Geometry check sheet. Reference: the model listing, model coordinates, mm. A direction names the side the tool comes from. Give positions to 0.01 mm unless a question says otherwise; leave off trailing zeros. Write each loop counter-clockwise with the first axis right and the second up, starting at its lowest first coordinate (ties: lowest second). Pieces come first, ordered by that corner, then holes. Notation, with made-up numbers: (27, 44) - (82, 44) arc R15 ccw to (82, 64) - close; hole circle Ø1 at (2, 4.5). An arc over 180 degrees is marked (long way). Write item = value, one per line. Start each with the question number.
(1) Section check D-D, the plane x = 12.5. Enter the section's corners in (y, z), plus the area to 3 significant figures.
(2) Depth check by flat-ended pin: pin 1 Ø8 at (x, z) = (-5.5, 4) entering from +Y; pin 2 Ø6 at (y, z) = (-4, 3.5) entering from -X; pin 3 Ø5 at (x, z) = (-17, 3.5) entering from -Y. Enter the tip coordinate at first touch or a pass-through.
(3) Section check C-C, the plane z = 0.75. Enter the section's corners in (x, y) (3 decimals), plus the area to 3 significant figures.
(4) Draft check along X on faces 1 (the flat face through (0, 0, 10.81)), 2 (the cylindrical face through (4.82, 7.063, 3.602)), 3 (the cylindrical face through (5.373, -40.924, 0.053)). Enter one of: pulls with the +X half, pulls with the -X half, needs draft (parallel to the pull), parting line crosses it, or undercut.
(5) Section check B-B, the plane x = -5.08. Enter the section's corners in (y, z).
(6) Thickness scan on L1, parallel to Y at x = -4, z = 1.75; L2, parallel to Z at x = 35.5, y = 11.5; L3, parallel to Y at x = -0.5, z = 1. Record the ranges inside material, lowest first.
(7) Access from +Z, -Z, +X, -X, +Y, -Y to the whole of each face (thin tool, end or side, straight path). Record for faces 4 (the cylindrical face through (9.237, -3.83, 7.261)), 5 (the cylindrical face through (-6.155, -6.766, 3.602)).
(8) Section check A-A, the plane y = 0. Enter the section's corners in (x, z) (3 decimals), plus the area to 3 significant figures.
```python
from build123d import *

# Parameters (mm, degrees)
SKETCH5_R           = 41.275
BOSS_EXTRUDE1_DEPTH = 3.81
SKETCH7_R           = 9.999849952
BOSS_EXTRUDE2_DEPTH = 7
SKETCH8_R           = 2
CUT_EXTRUDE1_DEPTH  = 61.174709389
CIRPATTERN1_COUNT   = 4


with BuildPart() as part:
    # Sketch5 → Boss-Extrude1 (new, symmetric)
    with BuildSketch(Plane.XY):
        with Locations(Location((0, 0, 0), (0, 0, 180))):
            Circle(SKETCH5_R)
    extrude(amount=BOSS_EXTRUDE1_DEPTH, both=True)

    # Sketch7 → Boss-Extrude2 (add)
    with BuildSketch(Plane.XY.offset(3.81)):
        Circle(SKETCH7_R)
    extrude(amount=BOSS_EXTRUDE2_DEPTH)

    # Sketch8 → Cut-Extrude1 (cut, through all)
    with BuildSketch(Plane.XY.offset(10.81)):
        with Locations((5.08, 5.08)):
            Circle(SKETCH8_R)
    cut_extrude1 = extrude(amount=-CUT_EXTRUDE1_DEPTH, mode=Mode.SUBTRACT)

    # CirPattern1: Cut-Extrude1 ×4 about axis
    cirpattern1_axis = Axis((0, 0, 0), (0, 0, 1))
    for i in range(1, CIRPATTERN1_COUNT):
        add(cut_extrude1.rotate(cirpattern1_axis, i * 360 / CIRPATTERN1_COUNT), mode=Mode.SUBTRACT)


solid = part.part
```
Model answer:
q1.outline = (-39.34, -3.81) - (39.34, -3.81) - (39.34, 3.81) - (-39.34, 3.81) - close
q1.area = 599 mm²
q2.pin_1 = 41.25
q2.pin_2 = -41.26
q2.pin_3 = -38.64
q3.outline = circle Ø82.55 at (0, 0); hole circle Ø4 at (-5.08, -5.08); hole circle Ø4 at (-5.08, 5.08); hole circle Ø4 at (5.08, -5.08); hole circle Ø4 at (5.08, 5.08)
q3.area = 5,300 mm²
q4.face_1 = needs draft
q4.face_2 = undercut
q4.face_3 = parting line crosses it
q5.outline = (-40.96, -3.81) - (-7.08, -3.81) - (-7.08, 10.81) - (-8.61, 10.81) - (-8.61, 3.81) - (-40.96, 3.81) - close; (-3.08, -3.81) - (3.08, -3.81) - (3.08, 10.81) - (-3.08, 10.81) - close; (7.08, -3.81) - (40.96, -3.81) - (40.96, 3.81) - (8.61, 3.81) - (8.61, 10.81) - (7.08, 10.81) - close
q6.L1 = -41.08 to -6.76, -3.4 to 3.4, 6.76 to 41.08
q6.L2 = -3.81 to 3.81
q6.L3 = -41.27 to 41.27
q7.face_4 = +Z
q7.face_5 = +Z, -Z
q8.outline = (-41.275, -3.81) - (41.275, -3.81) - (41.275, 3.81) - (10, 3.81) - (10, 10.81) - (-10, 10.81) - (-10, 3.81) - (-41.275, 3.81) - close
q8.area = 769 mm²
